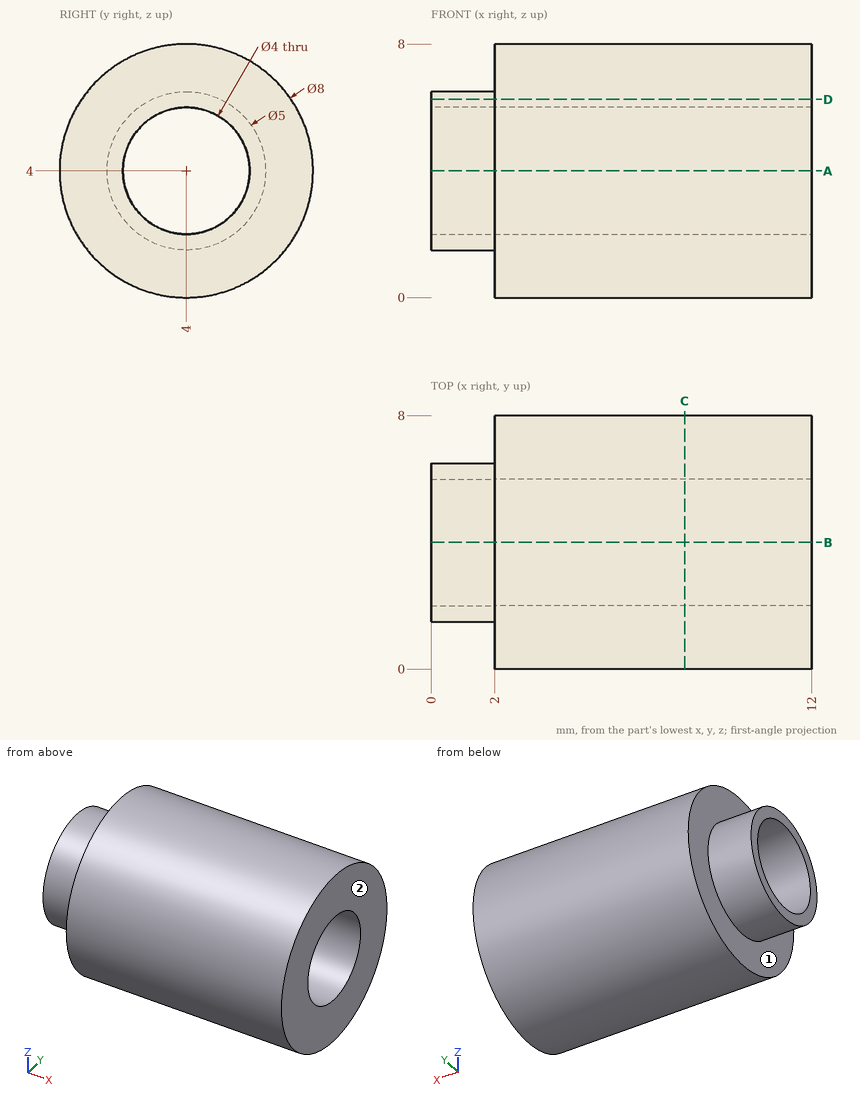
Answer from the drawing. Dimensions are ordinates in mm from the lowest x, y and z of the part. A direction names the side the tool comes from. Round coordinates to 2 decimals unless told otherwise and drop trailing zeros. Write each loop counter-clockwise with the first axis right and the second up, starting at its lowest first coordinate (ties: lowest second). Pieces come first, ordered by that corner, then holes. Notation, with made-up numbers: (-27, -26.5) - (19, -26.5) arc R24 ccw to (19, -14.5) - close; hole circle Ø11 at (6.5, -28). An arc over 180 degrees is marked (long way). One line per item, written item: value.
Q1. Find section D-D (z = 6.25). Determine the outline of the cut face in (x, y).
The answers:
outline: (0, 2.91) - (2, 2.91) - (2, 0.69) - (12, 0.69) - (12, 7.31) - (2, 7.31) - (2, 5.09) - (0, 5.09) - close
Q2. Straight lines are drawn through the part: line 1 (Y direction, x = 7.5, z = 4); line 2 (Y direction, x = 1.2, z = 4); line 3 (X direction, y = 3.75, z = 0.5). For each, find the intervals that lie inside material, in ascending order. Write a range as from..to.
The answers:
line 1: y = 0..2, 6..8
line 2: y = 1.5..2, 6..6.5
line 3: x = 2..12
Q3. Which of the six approach directions +Z, -Z, +X, -X, +Y, -Y give full straight-line access (tool end or side, diameter ignored) to the marked faces 1 and 2?
The answers:
face 1: -X
face 2: +Z, -Z, +X, +Y, -Y
Q4. Find section A-A (z = 4). Determine the outline of the cut face in (x, y).
The answers:
outline: (0, 1.5) - (2, 1.5) - (2, 0) - (12, 0) - (12, 2) - (0, 2) - close; (0, 6) - (12, 6) - (12, 8) - (2, 8) - (2, 6.5) - (0, 6.5) - close
Q5. Find section C-C (x = 8). Determine the outline of the cut face in (y, z), and give its area (3 significant figures).
The answers:
outline: circle Ø8 at (4, 4); hole circle Ø4 at (4, 4)
area: 37.7 mm2
